The model under review builds one solid part; all positions refer to its coordinate system, in mm. A direction names the side the tool comes from. Round coordinates to 2 decimals unless told otherwise and drop trailing zeros. Order: outer loops, then holes, each group sorted by start corner. A loop starts at its lowest first (then second) coordinate and runs counter-clockwise, first axis right, second up. Notation, with made-up numbers: (12.5, -39) - (67.5, -39) arc R18 cw to (67.5, -9) - close; hole circle Ø4 at (11.25, -11.5). An arc over 180 degrees is marked (long way). One line per question, with ' | ' between items. Start each with the question number.
Item 1: Draft analysis for pull direction Y (two halves, no side actions). For faces 1 (the face through (-20, 29, 2)), 2 (the face through (0, 57, 2)), 3 (the face through (0, 47, 2)), state which applies: +Y half, -Y half, draft (parallel to the pull), parting line (faces both ways), or undercut.
Item 2: For L1, parallel to Y at x = 0, z = 3.9; L2, parallel to Y at x = 17, z = 2.95; L3, parallel to Y at x = -3.5, z = 4.1, list the stretches that pass through material, from the lowest coordinate up. Write a range as [from, to].
Item 3: Insertion check: pin 1 Ø1.5 at (x, z) = (18, 2.5) entering from -Y; pin 2 Ø1.5 at (x, z) = (-17.5, 3.5) entering from -Y; pin 3 Ø1.5 at (x, z) = (18.5, 1.5) entering from -Y. Each pin has a flat end and moves straight along its axis. Give the tip position at first contact, or say it passes through.
Item 4: Tool access review of faces 4 (the face through (-18, 51, 2)), 5 (the face through (17, 11, 2)), 6 (the face through (-5, 29, 5)): name each direction out of +Z, -Z, +X, -X, +Y, -Y from which nothing blocks a thin tool from reaching the whole face with its end or side.
Item 5: Add section C-C on z = 4.4. State the section outline as (x, y) points.
Item 6: Add section D-D on y = 28.5. State the section outline as (x, z) points.
Item 7: Add section B-B on x = 0. State the section outline as (y, z) points.
Item 8: Add section A-A on y = 8.5. State the section outline as (x, z) points.
from build123d import *

# Parameters (mm, degrees)
ESQUISSE1_R        = 1.5
ESQUISSE1_R_2      = 4.25
BOSS_EXTRU_1_DEPTH = 5
CONG_1_R           = 5


with BuildPart() as part:
    # Esquisse1 → Boss.-Extru.1 (new body)
    with BuildSketch(Plane.XY):
        Polygon((-20, 0), (20, 0), (20, 6), (15, 6), (15, 11), (20, 11), (20, 46), (15, 46), (15, 51), (20, 51), (20, 57), (-20, 57), (-20, 51), (-15, 51), (-15, 46), (-20, 46), (-20, 11), (-15, 11), (-15, 6), (-20, 6), align=None)
        with Locations((0, 48.5)):
            Circle(ESQUISSE1_R, mode=Mode.SUBTRACT)
        with Locations((0, 8.5)):
            Circle(ESQUISSE1_R, mode=Mode.SUBTRACT)
        with Locations((0, 28.5)):
            Circle(ESQUISSE1_R_2, mode=Mode.SUBTRACT)
    extrude(amount=BOSS_EXTRU_1_DEPTH)

    # Congé1
    cong_1_edges = [part.edges().sort_by_distance(p)[0] for p in [
        (-20, 57, 2.5),
        (20, 57, 2.5),
        (20, 0, 2.5),
        (-20, 0, 2.5),
    ]]
    fillet(cong_1_edges, radius=CONG_1_R)


solid = part.part
Determined:
1) face 1: draft | face 2: +Y half | face 3: undercut
2) L1: [0, 7], [10, 24.25], [32.75, 47], [50, 57] | L2: [0.42, 6], [11, 46], [51, 56.58] | L3: [0, 26.09], [30.91, 57]
3) pin 1: y = 0.53 | pin 2: y = 0.32 | pin 3: y = 0.82
4) face 4: +Z, -Z, -X | face 5: +Z, -Z, +X | face 6: +Z, +X, -X, +Y, -Y
5) outline: (-20, 5) arc R5 ccw to (-15, 0) - (15, 0) arc R5 ccw to (20, 5) - (20, 6) - (15, 6) - (15, 11) - (20, 11) - (20, 46) - (15, 46) - (15, 51) - (20, 51) - (20, 52) arc R5 ccw to (15, 57) - (-15, 57) arc R5 ccw to (-20, 52) - (-20, 51) - (-15, 51) - (-15, 46) - (-20, 46) - (-20, 11) - (-15, 11) - (-15, 6) - (-20, 6) - close; hole circle Ø8.5 at (0, 28.5); hole circle Ø3 at (0, 8.5); hole circle Ø3 at (0, 48.5)
6) outline: (-20, 0) - (-4.25, 0) - (-4.25, 5) - (-20, 5) - close; (4.25, 0) - (20, 0) - (20, 5) - (4.25, 5) - close
7) outline: (0, 0) - (7, 0) - (7, 5) - (0, 5) - close; (10, 0) - (24.25, 0) - (24.25, 5) - (10, 5) - close; (32.75, 0) - (47, 0) - (47, 5) - (32.75, 5) - close; (50, 0) - (57, 0) - (57, 5) - (50, 5) - close
8) outline: (-15, 0) - (-1.5, 0) - (-1.5, 5) - (-15, 5) - close; (1.5, 0) - (15, 0) - (15, 5) - (1.5, 5) - close
